```python
from build123d import *

# Parameters (mm, degrees)
SKIZZE3_R                            = 3
SKIZZE3_R_2                          = 2
AUFSATZ_LINEAR_AUSTRAGEN1_DEPTH      = 3
AUFSATZ_LINEAR_AUSTRAGEN1_DEPTH_BACK = 3


with BuildPart() as part:
    # Skizze3 → Aufsatz-Linear austragen1 (new body, two sides)
    with BuildSketch(Plane.XY) as aufsatz_linear_austragen1_sk:
        with BuildLine():
            Line((24.349022765, 567.935323067), (65.349022765, 671.835323067))
            ThreePointArc((65.349022765, 671.835323067), (71.835323067, 674.650977235), (74.650977235, 668.164676933))
            Line((74.650977235, 668.164676933), (33.650977235, 564.264676933))
            ThreePointArc((33.650977235, 564.264676933), (27.164676933, 561.449022765), (24.349022765, 567.935323067))
        make_face()
        with Locations((70, 670)):
            Circle(SKIZZE3_R, mode=Mode.SUBTRACT)
        with Locations((29, 566.1)):
            Circle(SKIZZE3_R_2, mode=Mode.SUBTRACT)
    extrude(amount=AUFSATZ_LINEAR_AUSTRAGEN1_DEPTH)
    extrude(aufsatz_linear_austragen1_sk.sketch, amount=-AUFSATZ_LINEAR_AUSTRAGEN1_DEPTH_BACK)


solid = part.part
```
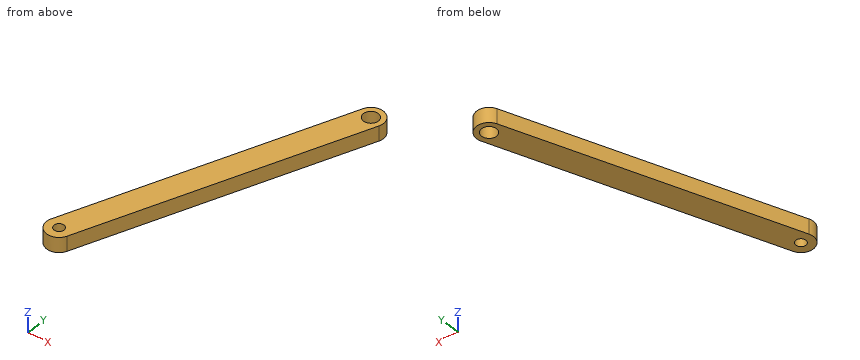
Geometry check sheet. Reference: the model listing, model coordinates, mm. Coordinates: 2 decimals unless noted, no trailing zeros. Order: outer loops, then holes, each group sorted by start corner. A loop starts at its lowest first (then second) coordinate and runs counter-clockwise, first axis right, second up.
Q1. Thickness scan on probe 1 along X at (y, z) = (566.1, -0.7); probe 2 along X at (y, z) = (670, -1.4); probe 3 along X at (y, z) = (614, 1.9). Record the ranges inside material, lowest first.
Reply:
probe 1: x = 24 to 27, 31 to 34.38
probe 2: x = 64.62 to 67, 73 to 75
probe 3: x = 42.53 to 53.28
Q2. Sectioned sample at D-D on y = 644.5. Record the cut outline in (x, z).
Reply:
outline: (54.56, -3) - (65.31, -3) - (65.31, 3) - (54.56, 3) - close
Q3. Sectioned sample at A-A on z = 0.25. Record the cut outline in (x, y), and give its area (3 significant figures).
Reply:
outline: (24.35, 567.94) arc R5 ccw to (33.65, 564.26) - (74.65, 668.16) arc R5 ccw to (65.35, 671.84) - close; hole circle Ø4 at (29, 566.1); hole circle Ø6 at (70, 670)
area: 1,150 mm2
Q4. Depth check by flat-ended pin: pin 1 Ø1.5 at (y, z) = (596, 2.5) entering from -X; pin 2 Ø5.5 at (x, y) = (70, 670) entering from -Z; pin 3 Ø2 at (y, z) = (576, -0.5) entering from +X. Enter the tip coordinate at first touch or a pass-through.
Reply:
pin 1: stops at x = 35.13
pin 2: passes through
pin 3: stops at x = 38.68
Q5. Sectioned sample at B-B on x = 29. Record the cut outline in (y, z), and give its area (3 significant figures).
Reply:
outline: (561.1, -3) - (564.1, -3) - (564.1, 3) - (561.1, 3) - close; (568.1, -3) - (579.72, -3) - (579.72, 3) - (568.1, 3) - close
area: 87.7 mm2
Q6. Sectioned sample at C-C on y = 566.1. Record the cut outline in (x, z), and give its area (3 significant figures).
Reply:
outline: (24, -3) - (27, -3) - (27, 3) - (24, 3) - close; (31, -3) - (34.38, -3) - (34.38, 3) - (31, 3) - close
area: 38.3 mm2
